Part model, mm, in its own coordinate system. Face numbers are marked on the shaded views. Coordinates: 2 decimals unless noted, no trailing zeros. Order: outer loops, then holes, each group sorted by start corner. A loop starts at its lowest first (then second) coordinate and runs counter-clockwise, first axis right, second up.
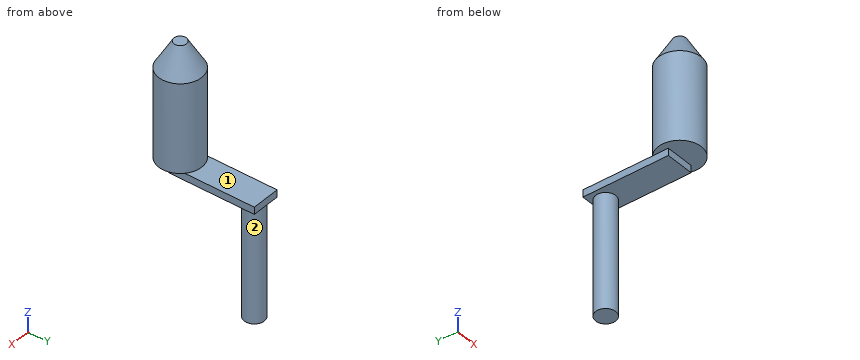
from build123d import *

# Parameters (mm, degrees)
SKETCH1_R           = 9.525
BOSS_EXTRUDE1_DEPTH = 50.8
SKETCH2_W           = 12.7
SKETCH2_H           = 38.1
BOSS_EXTRUDE2_DEPTH = 3.175
SKETCH3_R           = 4.445
BOSS_EXTRUDE3_DEPTH = 50.8


with BuildPart() as part:
    # Sketch1 → Boss-Extrude1 (new body)
    with BuildSketch(Plane.XY):
        Circle(SKETCH1_R)
    extrude(amount=BOSS_EXTRUDE1_DEPTH)

    # Sketch2 → Boss-Extrude2 (add)
    with BuildSketch(Plane(origin=(0, 0, 0), x_dir=(-1, 0, 0), z_dir=(0, 0, -1))):
        with Locations((0, 19.05)):
            Rectangle(SKETCH2_W, SKETCH2_H)
    extrude(amount=BOSS_EXTRUDE2_DEPTH)

    # Sketch3 → Boss-Extrude3 (add)
    with BuildSketch(Plane(origin=(0, 0, -3.175), x_dir=(-1, 0, 0), z_dir=(0, 0, -1))):
        with Locations(Location((0, 33.02, 0), (0, 0, 180))):
            Circle(SKETCH3_R)
    extrude(amount=BOSS_EXTRUDE3_DEPTH)

    # Sketch4 → Cut-Revolve1 (revolve, cut)
    with BuildSketch(Plane(origin=(0, 0, 0), x_dir=(0, 0, -1), z_dir=(1, 0, 0)), mode=Mode.PRIVATE) as cut_revolve1_sk:
        Polygon((-50.8, 2.77134643), (-39.232133446, 9.525), (-50.8, 9.525), align=None)
    revolve(cut_revolve1_sk.sketch.rotate(Axis((0, 0, -0.789350743), (0, 0, 1)), 90), axis=Axis((0, 0, -0.789350743), (0, 0, 1)), mode=Mode.SUBTRACT)


solid = part.part
Q1. Cut at C-C on y = 22.5. Write the cut outline in (x, z) (3 decimals), and give its area (3 significant figures).
Results list:
outline: (-6.35, -3.175) - (6.35, -3.175) - (6.35, 0) - (-6.35, 0) - close
area: 40.3 mm2
Q2. Mould opens along Y. For the marked faces 1 and 2 say: pulls with the +Y half, pulls with the -Y half, needs draft (parallel to the pull), parting line crosses it, or undercut.
Results list:
face 1: needs draft
face 2: parting line crosses it
Q3. Pin check, flat tips, straight feed: pin 1 Ø1 at (x, z) = (-1, -1.5) entering from -Y; pin 2 Ø8 at (x, z) = (-6.5, 36.5) entering from -Y; pin 3 Ø1 at (y, z) = (23, -1) entering from +X; pin 4 Ø10 at (y, z) = (-3, 37) entering from -X (3 decimals). Stop position of each tip, or through.
Results list:
pin 1: stops at y = 0
pin 2: stops at y = -9.19
pin 3: stops at x = 6.35
pin 4: stops at x = -9.525
Q4. Wall check: line 1 along Y through (x, z) = (0, 21.5) (3 decimals); line 2 along Z through (x, y) = (4.75, 33.5) (3 decimals); line 3 along Y through (x, z) = (0, -4) (3 decimals). Give the ranges that are in metal, low to high.
Results list:
line 1: y = -9.525 to 9.525
line 2: z = -3.175 to 0
line 3: y = 28.575 to 37.465
Q5. Cut at D-D on z = 10. Write the cut outline in (x, y) (3 decimals), and give its area (3 significant figures).
Results list:
outline: circle Ø19.05 at (0, 0)
area: 285 mm2
Q6. Cut at A-A on x = 0. Write the cut outline in (y, z) (3 decimals), and give its area (3 significant figures).
Results list:
outline: (-9.525, 0) - (0, 0) - (0, -3.175) - (28.575, -3.175) - (28.575, -53.975) - (37.465, -53.975) - (37.465, -3.175) - (38.1, -3.175) - (38.1, 0) - (9.525, 0) - (9.525, 39.232) - (2.771, 50.8) - (-2.771, 50.8) - (-9.525, 39.232) - close
area: 1,460 mm2
Q7. Cut at B-B on z = -38. Write the cut outline in (x, y) (3 decimals), and give its area (3 significant figures).
Results list:
outline: circle Ø8.89 at (0, 33.02)
area: 62.1 mm2
